from build123d import *

# Parameters (mm, degrees)
SKETCH1_W           = 45.72
SKETCH1_H           = 81.28
BOSS_EXTRUDE1_DEPTH = 7.62
SKETCH7_W           = 40.64
SKETCH7_H           = 81.28
BOSS_EXTRUDE3_DEPTH = 5.08
SKETCH8_W           = 40.64
SKETCH8_H           = 81.28
BOSS_EXTRUDE4_DEPTH = 5.08
SKETCH9_W           = 55.88
SKETCH9_H           = 40.64
BOSS_EXTRUDE5_DEPTH = 5.08
SKETCH10_W          = 55.88
SKETCH10_H          = 40.64
BOSS_EXTRUDE6_DEPTH = 5.08


with BuildPart() as part:
    # Sketch1 → Boss-Extrude1 (new body)
    with BuildSketch(Plane.XY):
        with Locations((-26.67, -9.68375)):
            Rectangle(SKETCH1_W, SKETCH1_H)
    extrude(amount=BOSS_EXTRUDE1_DEPTH)

    # Sketch7 → Boss-Extrude3 (add)
    with BuildSketch(Plane.ZY.offset(49.53)):
        with Locations((-12.7, -9.68375)):
            Rectangle(SKETCH7_W, SKETCH7_H)
    extrude(amount=BOSS_EXTRUDE3_DEPTH)

    # Sketch8 → Boss-Extrude4 (add)
    with BuildSketch(Plane(origin=(-3.81, 0, 0), x_dir=(0, 0, -1), z_dir=(1, 0, 0))):
        with Locations((12.7, -9.68375)):
            Rectangle(SKETCH8_W, SKETCH8_H)
    extrude(amount=BOSS_EXTRUDE4_DEPTH)

    # Sketch9 → Boss-Extrude5 (add)
    with BuildSketch(Plane(origin=(0, 30.95625, 0), x_dir=(1, 0, 0), z_dir=(0, 1, 0))):
        with Locations((-26.67, 12.7)):
            Rectangle(SKETCH9_W, SKETCH9_H)
    extrude(amount=BOSS_EXTRUDE5_DEPTH)

    # Sketch10 → Boss-Extrude6 (add)
    with BuildSketch(Plane.XZ.offset(50.32375)):
        with Locations((-26.67, -12.7)):
            Rectangle(SKETCH10_W, SKETCH10_H)
    extrude(amount=BOSS_EXTRUDE6_DEPTH)


solid = part.part
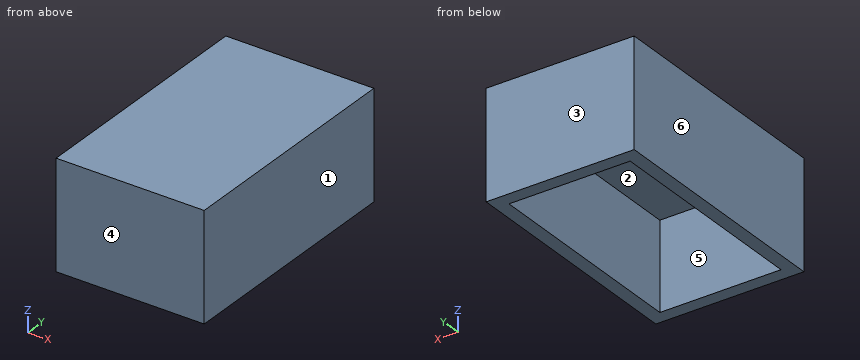
Design review of the part built by this model. Coordinates are the model's own, in mm. Face numbers are marked on the shaded views. A direction names the side the tool comes from. Give positions to 0.01 mm unless a question says otherwise; leave off trailing zeros. Loops run counter-clockwise (first coordinate to the right, second up) from the corner with the lowest first, then second, coordinate; pieces in that order, holes last. Notation, with made-up numbers: M 58.25,11 L 67.25,11 A33 cw 67.25,42 Z; hole C -6,-12.75 d2. An arc over 180 degrees is marked long. Write item = value, one per line.
Q1. We need section B-B (z = -15). Give the boundary of the cut face in (x, y).
Output values:
outline = M -54.61,-55.4 L 1.27,-55.4 L 1.27,36.04 L -54.61,36.04 Z; hole M -49.53,-50.32 L -3.81,-50.32 L -3.81,30.96 L -49.53,30.96 Z
Q2. For the marked faces 1 and 2, list the 3-axis set-ups (+Z, -Z, +X, -X, +Y, -Y) from which the entire face can be reached by the end or side of a thin tool; tool diameter is ignored.
Output values:
face_1 = +Z, -Z, +X, +Y, -Y
face_2 = -Z
Q3. We need section C-C (y = -15.5). Give the boundary of the cut face in (x, z).
Output values:
outline = M -54.61,-33.02 L -49.53,-33.02 L -49.53,0 L -3.81,0 L -3.81,-33.02 L 1.27,-33.02 L 1.27,7.62 L -54.61,7.62 Z
Q4. Insertion check: pin 1 (10 mm diameter, centred on x = -39.5, y = 12, fed in from -Z). The pin has a flat end and moves straight along its axis. Give the tip position at first contact, or say it passes through.
Output values:
pin_1 = 0
Q5. Draft analysis for pull direction Y (two halves, no side actions). For the marked faces 3, 4, 5 and 6, state which applies: +Y half, -Y half, draft (parallel to the pull), parting line (faces both ways), or undercut.
Output values:
face_3 = +Y half
face_4 = -Y half
face_5 = undercut
face_6 = draft
Q6. To check wall thickness, follow line 1 (X direction, y = 15.5, z = -22.5); line 2 (Y direction, x = -25, z = -5.5); line 3 (Z direction, x = -33.5, y = -22). State the ranges of each line that lie inside material, in increasing order. Write a range as [from, to].
Output values:
line_1 = [-54.61, -49.53], [-3.81, 1.27]
line_2 = [-55.4, -50.32], [30.96, 36.04]
line_3 = [0, 7.62]
Q7. We need section A-A (x = -39). Give the boundary of the cut face in (y, z), plus the area to 3 significant figures.
Output values:
outline = M -55.4,-33.02 L -50.32,-33.02 L -50.32,0 L 30.96,0 L 30.96,-33.02 L 36.04,-33.02 L 36.04,7.62 L -55.4,7.62 Z
area = 1,030 mm^2
